from build123d import *

# Parameters (mm, degrees)
SZKIC2_R                    = 2.3
DODANIE_WYCI_GNI_CIE1_DEPTH = 4
SZKIC3_R                    = 1.75
DODANIE_WYCI_GNI_CIE2_DEPTH = 17
DODANIE_WYCI_GNI_CIE3_DEPTH = 14
SZKIC6_R                    = 2.3
SZKIC6_R_2                  = 1.75
WYTNIJ_WYCI_GNI_CIE2_DEPTH  = 131.905876654


with BuildPart() as part:
    # Szkic2 → Dodanie-wyciągnięcie1 (new body)
    with BuildSketch(Plane.XY):
        with BuildLine():
            Line((15.2, 17.1), (15.2, 10.1))
            Line((15.2, 10.1), (20.2, 10.1))
            Line((20.2, 10.1), (20.2, -10.1))
            Line((20.2, -10.1), (15.2, -10.1))
            Line((15.2, -10.1), (15.2, -17.1))
            Line((15.2, -17.1), (19.197379501, -17.1))
            ThreePointArc((19.197379501, -17.1), (72.757727431, -17.908543704), (126.269263581, -20.333437957))
            ThreePointArc((126.269263581, -20.333437957), (127.600370297, -18.154974458), (126.216652739, -16.009543491))
            ThreePointArc((126.216652739, -16.009543491), (78.887653554, 2.515256091), (30.2, 17.1))
            Line((30.2, 17.1), (15.2, 17.1))
        make_face()
        with Locations(Location((25.2, 4.6, 0), (0, 0, 180))):
            Circle(SZKIC2_R, mode=Mode.SUBTRACT)
        with Locations((25.2, -4.6)):
            Circle(SZKIC2_R, mode=Mode.SUBTRACT)
    extrude(amount=DODANIE_WYCI_GNI_CIE1_DEPTH)

    # Szkic3 → Dodanie-wyciągnięcie2 (add)
    with BuildSketch(Plane.XY.offset(4)):
        with BuildLine():
            ThreePointArc((126.269263581, -20.333437957), (121.801544753, -20.069007105), (117.33317317, -19.815845914))
            ThreePointArc((117.33317317, -19.815845914), (116.687057134, -16.008461108), (118.922411718, -12.859360463))
            ThreePointArc((118.922411718, -12.859360463), (122.574580097, -14.42276365), (126.216652739, -16.009543491))
            ThreePointArc((126.216652739, -16.009543491), (127.600370297, -18.154974458), (126.269263581, -20.333437957))
        make_face()
        with Locations((121.2, -17.133437957)):
            Circle(SZKIC3_R, mode=Mode.SUBTRACT)
    extrude(amount=DODANIE_WYCI_GNI_CIE2_DEPTH)

    # Szkic5 → Dodanie-wyciągnięcie3 (add)
    with BuildSketch(Plane.XY.offset(4)):
        with BuildLine():
            Line((20.5, -4.6), (20.5, 4.6))
            ThreePointArc((20.5, 4.6), (25.2, 9.3), (29.9, 4.6))
            Line((29.9, 4.6), (29.9, -4.6))
            ThreePointArc((29.9, -4.6), (25.2, -9.3), (20.5, -4.6))
        make_face()
    extrude(amount=DODANIE_WYCI_GNI_CIE3_DEPTH)

    # Szkic6 → Wytnij-wyciągnięcie2 (cut, through all)
    with BuildSketch(Plane(origin=(0, 0, 0), x_dir=(-1, 0, 0), z_dir=(0, 0, -1))):
        with Locations(Location((-25.2, -4.6, 0), (0, 0, 180))):
            Circle(SZKIC6_R)
        with Locations((-25.2, 4.6)):
            Circle(SZKIC6_R)
        with Locations((-121.2, -17.133437957)):
            Circle(SZKIC6_R_2)
    extrude(amount=-WYTNIJ_WYCI_GNI_CIE2_DEPTH, mode=Mode.SUBTRACT)


solid = part.part
For this review, take the finished solid that the model builds, in its own axes (mm). A direction names the side the tool comes from. Round coordinates to 2 decimals unless told otherwise and drop trailing zeros. Write each loop counter-clockwise with the first axis right and the second up, starting at its lowest first coordinate (ties: lowest second). Pieces come first, ordered by that corner, then holes. Notation, with made-up numbers: (89.25, 84.5) -> (121.25, 84.5) arc R22 ccw to (121.25, 111.5) -> close; hole circle Ø4 at (89.5, -30.75). An arc over 180 degrees is marked (long way). Put each result on its own line as item: value.
Q1. Machinability: for faces 1 (the cylindrical face through (25.3, -9.3, 10.9)), 2 (the flat face through (20.5, 0, 11)), 3 (the flat face through (18, 10.1, 2)), 4 (the cylindrical face through (116.675, -16.063, 12.381)), which of the approach directions +Z, -Z, +X, -X, +Y, -Y give a long, thin tool a straight path to every point of the face, cutting with its end or side? Answer none if there is none.
Determined:
face 1: +Z, -Y
face 2: +Z, -X, +Y, -Y
face 3: +Z, -Z, -X
face 4: +Z, -X
Q2. Clearance check with flat-ended pins moving along their axes: pin 1 Ø10 at (y, z) = (1.5, 11) entering from -X; pin 2 Ø1.2 at (x, z) = (17.5, 2) entering from -Y; pin 3 Ø4 at (y, z) = (5.5, 17.5) entering from +X. State where each tip first meets the part, or that it passes through.
Determined:
pin 1: stops at x = 20.5
pin 2: stops at y = -17.1
pin 3: stops at x = 29.9
Q3. Consider section A-A on x = 120.5. State the section outline as (y, z) points, and give its area (3 significant figures).
Determined:
outline: (-19.99, 0) -> (-18.74, 0) -> (-18.74, 21) -> (-19.99, 21) -> close; (-15.53, 0) -> (-13.53, 0) -> (-13.53, 21) -> (-15.53, 21) -> close
area: 68.4 mm^2
Q4. Consider section C-C on x = 25.2. State the section outline as (y, z) points, and give its area (3 significant figures).
Determined:
outline: (-17.11, 0) -> (-6.9, 0) -> (-6.9, 18) -> (-9.3, 18) -> (-9.3, 4) -> (-17.11, 4) -> close; (-2.3, 0) -> (2.3, 0) -> (2.3, 18) -> (-2.3, 18) -> close; (6.9, 0) -> (17.1, 0) -> (17.1, 4) -> (9.3, 4) -> (9.3, 18) -> (6.9, 18) -> close
area: 232 mm^2
Q5. Consider section D-D on y = 8. State the section outline as (x, z) points (3 decimals), and give its area (3 significant figures).
Determined:
outline: (20.2, 0) -> (62.22, 0) -> (62.22, 4) -> (28.445, 4) -> (28.445, 18) -> (21.955, 18) -> (21.955, 4) -> (20.2, 4) -> close
area: 259 mm^2
Q6. The part is to be moulded in two halves that separate along Y. For faces 5 (the flat face through (29.9, 0, 11)), 6 (the cylindrical face through (25.1, 9.3, 10.9)), 7 (the flat face through (17, -17.1, 2)), 8 (the flat face through (18, -10.1, 2)), say which applies: released by +Y, released by -Y, zero draft, split by the parting line, or undercut.
Determined:
face 5: zero draft
face 6: released by +Y
face 7: released by -Y
face 8: undercut
Q7. Consider section B-B on z = 7.25. State the section outline as (x, y) points, and give its area (3 significant figures).
Determined:
outline: (20.5, -4.6) arc R4.7 ccw to (29.9, -4.6) -> (29.9, 4.6) arc R4.7 ccw to (20.5, 4.6) -> close; (117.33, -19.82) arc R1774.4 cw to (126.27, -20.33) arc R2.4 ccw to (126.22, -16.01) arc R619.81 ccw to (118.92, -12.86) arc R5.05 ccw to start; hole circle Ø4.6 at (25.2, -4.6); hole circle Ø4.6 at (25.2, 4.6); hole circle Ø3.5 at (121.2, -17.13)
area: 172 mm^2
Q8. To check wall thickness, follow L1, parallel to Y at x = 25.2, z = 5.25; L2, parallel to X at y = -4.6, z = 10.5; L3, parallel to Z at x = 106.5, y = -8. State the ranges of each line that lie inside material, in increasing order. Write a range as [from, to].
Determined:
L1: y = [-9.3, -6.9], [-2.3, 2.3], [6.9, 9.3]
L2: x = [20.5, 22.9], [27.5, 29.9]
L3: z = [0, 4]
